Check sheet for the drawn part. Datum: minimum x, y, z corner. Units: mm. A direction names the side the tool comes from. Coordinates: 2 decimals unless noted, no trailing zeros. Write each loop counter-clockwise with the first axis right and the second up, starting at its lowest first coordinate (ties: lowest second). Pieces come first, ordered by that corner, then holes. Notation, with made-up numbers: (-17, -20) - (7, -20) arc R25 ccw to (7, 4) - close; hole circle Ø1 at (10.5, 4). An arc over 180 degrees is marked (long way). Write each question's results on one line, items separated by ' | '.
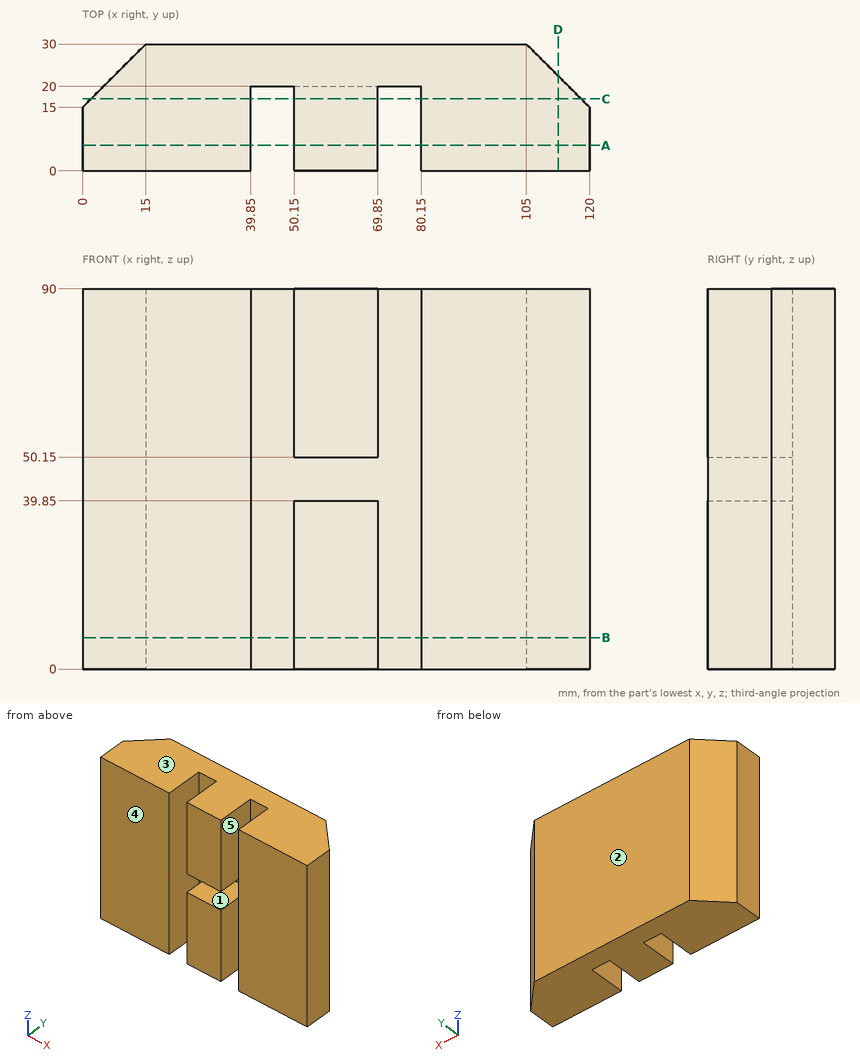
1. Sectioned sample at A-A (y = 6). Record the cut outline in (x, z), then the cut area to 3 significant figures.
Values follow:
outline: (0, 0) - (39.85, 0) - (39.85, 90) - (0, 90) - close; (50.15, 0) - (69.85, 0) - (69.85, 39.85) - (50.15, 39.85) - close; (50.15, 50.15) - (69.85, 50.15) - (69.85, 90) - (50.15, 90) - close; (80.15, 0) - (120, 0) - (120, 90) - (80.15, 90) - close | area: 8,740 mm^2
2. Go/stop test with flat-tipped pins: pin 1 (6 mm diameter, centred on y = 23, z = 81, fed in from -X); pin 2 (1 mm diameter, centred on y = 19, z = 63.5, fed in from -X). Record where each tip stops, or that it passes through.
Values follow:
pin 1: stops at x = 5 | pin 2: stops at x = 3.5
3. Draft check along Z on the marked faces 1, 2 and 3. Enter one of: pulls with the +Z half, pulls with the -Z half, needs draft (parallel to the pull), parting line crosses it, or undercut.
Values follow:
face 1: undercut | face 2: needs draft | face 3: pulls with the +Z half
4. Access from +Z, -Z, +X, -X, +Y, -Y to the whole of each face (thin tool, end or side, straight path). Record for the marked faces 4 and 5.
Values follow:
face 4: +Z, -Z, +X, -X, -Y | face 5: +Z, -Z, -Y
5. Sectioned sample at D-D (x = 112.5). Record the cut outline in (y, z).
Values follow:
outline: (0, 0) - (22.5, 0) - (22.5, 90) - (0, 90) - close
6. Sectioned sample at B-B (z = 7.5). Record the cut outline in (x, y), then the cut area to 3 significant figures.
Values follow:
outline: (0, 0) - (39.85, 0) - (39.85, 20) - (50.15, 20) - (50.15, 0) - (69.85, 0) - (69.85, 20) - (80.15, 20) - (80.15, 0) - (120, 0) - (120, 15) - (105, 30) - (15, 30) - (0, 15) - close | area: 2,960 mm^2
7. Material ranges on L1, parallel to X at y = 14, z = 60.5; L2, parallel to X at y = 19, z = 8; L3, parallel to Z at x = 56, y = 16.75, recorded low to high. Write a range as [from, to].
Values follow:
L1: x = [0, 39.85], [50.15, 69.85], [80.15, 120] | L2: x = [4, 39.85], [50.15, 69.85], [80.15, 116] | L3: z = [0, 39.85], [50.15, 90]
8. Sectioned sample at C-C (y = 17). Record the cut outline in (x, z).
Values follow:
outline: (2, 0) - (39.85, 0) - (39.85, 90) - (2, 90) - close; (50.15, 0) - (69.85, 0) - (69.85, 39.85) - (50.15, 39.85) - close; (50.15, 50.15) - (69.85, 50.15) - (69.85, 90) - (50.15, 90) - close; (80.15, 0) - (118, 0) - (118, 90) - (80.15, 90) - close
